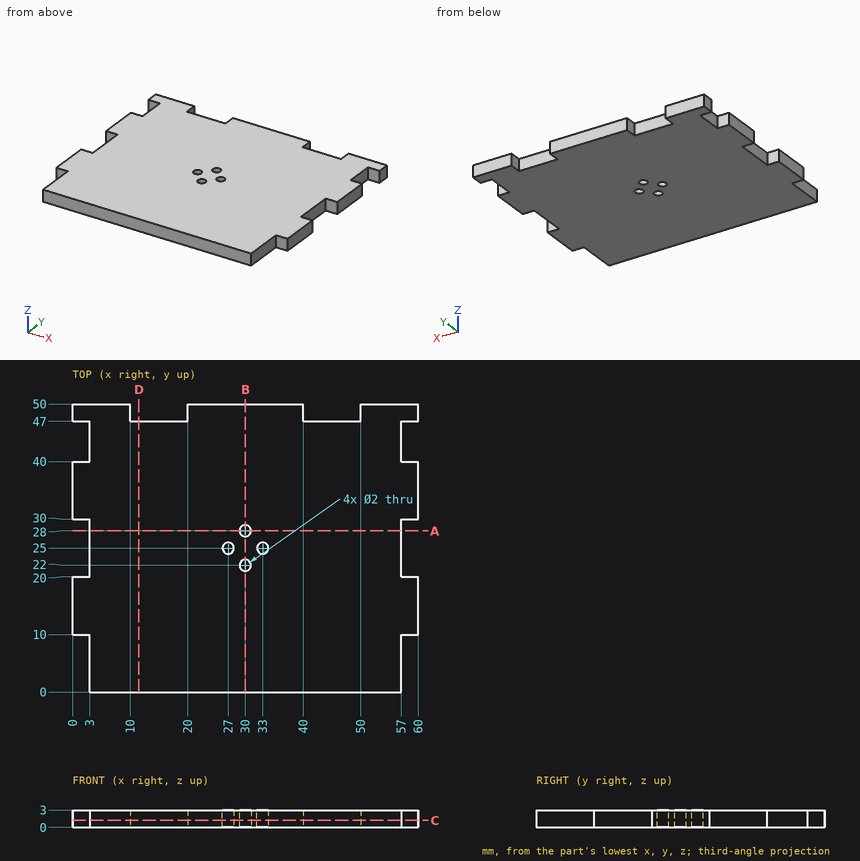
The figure shows three views and two pictorial views of one solid part (mm, origin at its lowest corner). Answer the questions. Round coordinates to 2 decimals unless told otherwise and drop trailing zeros. Write each loop counter-clockwise with the first axis right and the second up, starting at its lowest first coordinate (ties: lowest second). Pieces come first, ordered by that corner, then holes. Notation, with made-up numbers: (0.5, -12) - (8.5, -12) arc R21 cw to (8.5, 9) - close; hole circle Ø9 at (66.25, 9). An arc over 180 degrees is marked (long way). One line per question, with ' | ' between items. Start each with the question number.
1. Section C-C (z = 1.25) is taken. Give the number of separate pieces and of enclosed holes in the cut face, and give its area (3 significant figures).
2. Each of these flat-tipped pins is pushed along its axis until it touches: pin 1 (0.9 mm diameter, centred on y = 5, z = 1.5, fed in from +X); pin 2 (1.5 mm diameter, centred on x = 39, z = 0.5, fed in from -Y); pin 3 (1.8 mm diameter, centred on x = 30, y = 22, fed in from +Z). Where does it stop, or does it pass through?
3. Find the intervals of material crossed by probe 1 along Y at (x, z) = (30, 1); probe 2 along Y at (x, z) = (33, 1.05); probe 3 along X at (y, z) = (7, 1.7), in increasing order. Write a range as [from, to].
4. Section B-B (x = 30) is taken. Determine the outline of the cut face in (y, z).
5. Section A-A (y = 28) is taken. Determine the outline of the cut face in (x, z).
6. Section D-D (x = 11.5) is taken. Determine the outline of the cut face in (y, z).
Filled in:
1) separate pieces: 1 | enclosed holes: 4 | area: 2,770 mm²
2) pin 1: x = 57 | pin 2: y = 0 | pin 3: through
3) probe 1: [0, 21], [23, 27], [29, 50] | probe 2: [0, 24], [26, 50] | probe 3: [3, 57]
4) outline: (0, 0) - (21, 0) - (21, 3) - (0, 3) - close; (23, 0) - (27, 0) - (27, 3) - (23, 3) - close; (29, 0) - (50, 0) - (50, 3) - (29, 3) - close
5) outline: (3, 0) - (29, 0) - (29, 3) - (3, 3) - close; (31, 0) - (57, 0) - (57, 3) - (31, 3) - close
6) outline: (0, 0) - (47, 0) - (47, 3) - (0, 3) - close
